Part model, mm, in its own coordinate system. A direction names the side the tool comes from. Round coordinates to 2 decimals unless told otherwise and drop trailing zeros. Write each loop counter-clockwise with the first axis right and the second up, starting at its lowest first coordinate (ties: lowest second). Pieces come first, ordered by that corner, then holes.
```python
from build123d import *

# Parameters (mm, degrees)
F0_R           = 4
F1_DEPTH       = 14
F2_ANGLE       = 180
F4_D           = 5.5
F4_CSINK_D     = 6.5
F4_CSINK_ANGLE = 90


with BuildPart() as f1:
    # F0 (on Right) → F1 (new body)
    with BuildSketch(Plane.YZ):
        Polygon((-21, -19), (0, -19), (21, -19), (21, -13), (9, -13), (9, 14), (0, 14), (-9, 14), (-9, -13), (-21, -13), align=None)
        Circle(F0_R, mode=Mode.SUBTRACT)
    extrude(amount=F1_DEPTH)


with BuildPart() as f1_1:
    # F2: moved
    add(f1.part.rotate(Axis((0, 0, 0), (-1, 0, 0)), F2_ANGLE))

    # F4 (through all)
    with Locations(Plane.XY.offset(19)):
        with Locations((7, -16.25), (7, 16.25)):
            CounterSinkHole(F4_D / 2, F4_CSINK_D / 2, counter_sink_angle=F4_CSINK_ANGLE)


solid = f1_1.part
```
Q1. Cut at B-B on y = 16.25. Write the cut outline in (x, z).
Values follow:
outline: (0, 13) - (4.25, 13) - (4.25, 18.5) - (3.75, 19) - (0, 19) - close; (9.75, 13) - (14, 13) - (14, 19) - (10.25, 19) - (9.75, 18.5) - close
Q2. Cut at D-D on x = 7. Write the cut outline in (y, z), plus the area to 3 significant figures.
Values follow:
outline: (-21, 13) - (-19, 13) - (-19, 18.5) - (-19.5, 19) - (-21, 19) - close; (-13.5, 13) - (-9, 13) - (-9, -14) - (9, -14) - (9, 13) - (13.5, 13) - (13.5, 18.5) - (13, 19) - (-13, 19) - (-13.5, 18.5) - close; (19, 13) - (21, 13) - (21, 19) - (19.5, 19) - (19, 18.5) - close; hole circle Ø8 at (0, 0)
area: 621 mm2
Q3. Drop flat-ended pins along their axis: pin 1 (8 mm diameter, centred on x = 7.5, y = 13.5, fed in from -Z); pin 2 (4 mm diameter, centred on x = 9, z = 2.5, fed in from +Y); pin 3 (2 mm diameter, centred on x = 9, z = 4.5, fed in from -Y). Give the stop position or say it passes through.
Values follow:
pin 1: stops at z = 13
pin 2: stops at y = 9
pin 3: stops at y = -9
Q4. Which spindle directions (+Z, -Z, +X, -X, +Y, -Y) get a long thin tool onto all of the face, cutting with end or side? Do faces 4 (the flat face through (7, -9, 0)), 5 (the flat face through (7, 9, -1)), 6 (the flat face through (14, 0, 6)). Say none if no direction does.
Values follow:
face 4: -Z, +X, -X, -Y
face 5: -Z, +X, -X, +Y
face 6: +Z, -Z, +X, +Y, -Y
Q5. Cut at A-A on x = 12. Write the cut outline in (y, z), plus the area to 3 significant figures.
Values follow:
outline: (-21, 13) - (-9, 13) - (-9, -14) - (9, -14) - (9, 13) - (21, 13) - (21, 19) - (-21, 19) - close; hole circle Ø8 at (0, 0)
area: 688 mm2
Q6. Cut at C-C on z = 0. Write the cut outline in (x, y), plus the area to 3 significant figures.
Values follow:
outline: (0, -9) - (14, -9) - (14, -4) - (0, -4) - close; (0, 4) - (14, 4) - (14, 9) - (0, 9) - close
area: 140 mm2
Q7. Wall check: L1, parallel to Y at x = 7, z = 16; L2, parallel to Y at x = 10.75, z = 0; L3, parallel to Z at x = 11.25, y = 0. Give the ranges that are in metal, low to high.
Values follow:
L1: y = -21 to -19, -13.5 to 13.5, 19 to 21
L2: y = -9 to -4, 4 to 9
L3: z = -14 to -4, 4 to 19
Q8. Mould opens along Y. For faces 1 (the flat face through (8.5, 13.6, 13)), 2 (the cylindrical face through (4.38, -15.42, 15.71)), 3 (the flat face through (7, -21, 16)) say: +Y half, -Y half, draft (parallel to the pull), parting line (faces both ways), or undercut.
Values follow:
face 1: draft
face 2: undercut
face 3: -Y half
